CAD build for the part. Positions are in the model's coordinates, mm. A direction names the side the tool comes from. Coordinates: 2 decimals unless noted, no trailing zeros. Write each loop counter-clockwise with the first axis right and the second up, starting at its lowest first coordinate (ties: lowest second). Pieces come first, ordered by that corner, then holes. Notation, with made-up numbers: (54, 52) -> (72, 52) arc R20 cw to (72, 74) -> close; hole circle Ø1 at (44.5, -34.75). An arc over 180 degrees is marked (long way). Answer as CSV lines item,"result".
```python
from build123d import *

# Parameters (mm, degrees)
F0_R     = 5
F1_DEPTH = 4
F3_DEPTH = 12.5
F4_W     = 12
F4_H     = 12
F5_DEPTH = 3
F6_R     = 4.5
F7_DEPTH = 0.5


with BuildPart() as f1:
    # F0 (on Front) → F1 (new body)
    with BuildSketch(Plane.XZ):
        Circle(F0_R)
    extrude(amount=F1_DEPTH)

    # F2 (on Right) → F3 (cut, symmetric)
    with BuildSketch(Plane.YZ):
        Polygon((-5.130814, -6.028544), (-0.71682, -5.832574), (-4.290942, 0), align=None)
    extrude(amount=F3_DEPTH, both=True, mode=Mode.SUBTRACT)

    # F4 (on face) → F5 (join)
    with BuildSketch(Plane(origin=(0, 0, 0), x_dir=(-1, 0, 0), z_dir=(0, 1, 0))):
        Rectangle(F4_W, F4_H)
    extrude(amount=F5_DEPTH)

    # F6 (on face) → F7 (cut)
    with BuildSketch(Plane(origin=(0, 3, 0), x_dir=(-1, 0, 0), z_dir=(0, 1, 0))):
        Circle(F6_R)
    extrude(amount=-F7_DEPTH, mode=Mode.SUBTRACT)


solid = f1.part
```
Item 1: Flat gauge pins, fed straight in: pin 1 (2 mm diameter, centred on x = 3, z = -3.5, fed in from -Y); pin 2 (1 mm diameter, centred on x = 4, y = -1.5, fed in from +Z); pin 3 (2.5 mm diameter, centred on x = 1.5, z = -1.5, fed in from +Y). Where does each tip first touch, or does it go through?
Answer below:
pin 1,"stops at y = -2.76"
pin 2,"stops at z = 3.57"
pin 3,"stops at y = 2.5"
Item 2: 3-axis set-ups, long thin cutter, end or side, ignore diameter. For faces 4 (the flat face through (-5.2, 0, 0.1)), 5 (the flat face through (0, 2.5, 0)), 6 (the flat face through (-3, 3, 4)): which of +Z, -Z, +X, -X, +Y, -Y reach the whole face in a straight line?
Answer below:
face 4,"-Y"
face 5,"+Y"
face 6,"+Z, -Z, +X, -X, +Y"
Item 3: Saw through at B-B on x = 0. Give the cut face in (y, z).
Answer below:
outline,"(-4, -0.47) -> (-1.23, -5) -> (0, -5) -> (0, -6) -> (3, -6) -> (3, -4.5) -> (2.5, -4.5) -> (2.5, 4.5) -> (3, 4.5) -> (3, 6) -> (0, 6) -> (0, 5) -> (-4, 5) -> close"
Item 4: Saw through at A-A on z = 0. Give the cut face in (x, y).
Answer below:
outline,"(-6, 0) -> (-5, 0) -> (-5, -4) -> (5, -4) -> (5, 0) -> (6, 0) -> (6, 3) -> (4.5, 3) -> (4.5, 2.5) -> (-4.5, 2.5) -> (-4.5, 3) -> (-6, 3) -> close"
Item 5: Wall check: line 1 (Z direction, x = 0, y = 2.7); line 2 (Y direction, x = 5.25, z = 5.25); line 3 (Y direction, x = -1, z = 4). Give the ranges that are in metal, low to high. Write a range as from..to.
Answer below:
line 1,"z = -6..-4.5, 4.5..6"
line 2,"y = 0..3"
line 3,"y = -4..2.5"
Item 6: Saw through at C-C on y = 2.75. Give the cut face in (x, z), and give its area (3 significant figures).
Answer below:
outline,"(-6, -6) -> (6, -6) -> (6, 6) -> (-6, 6) -> close; hole circle Ø9 at (0, 0)"
area,"80.4 mm2"
Item 7: Two-plate mould, pull along Z, no slides. Class faces 1 (the cylindrical face through (0.59, 2.75, 4.46)), 2 (the cylindrical face through (-0.651, -1.528, 4.957)), 3 (the flat face through (0.07, -2.9, -2.27)): pulls with the +Z half, pulls with the -Z half, needs draft (parallel to the pull), parting line crosses it, or undercut.
Answer below:
face 1,"undercut"
face 2,"parting line crosses it"
face 3,"pulls with the -Z half"
Item 8: Saw through at D-D on z = -1.5. Give the cut face in (x, y), and give its area (3 significant figures).
Answer below:
outline,"(-6, 0) -> (-4.77, 0) -> (-4.77, -3.37) -> (4.77, -3.37) -> (4.77, 0) -> (6, 0) -> (6, 3) -> (4.24, 3) -> (4.24, 2.5) -> (-4.24, 2.5) -> (-4.24, 3) -> (-6, 3) -> close"
area,"63.9 mm2"
